from build123d import *

# Parameters (mm, degrees)
EXTRUDE_1_DEPTH = 0.5
SKETCH_2_W      = 15
SKETCH_2_H      = 2
EXTRUDE_2_DEPTH = 3.6


with BuildPart() as part:
    # 草圖1 → 填料-伸長1 (new body, symmetric)
    with BuildSketch(Plane.XY):
        with BuildLine():
            Line((-17.6, 110.46), (17.6, 110.46))
            ThreePointArc((17.6, 110.46), (26.056997103, 106.956997103), (29.56, 98.5))
            Line((29.56, 98.5), (29.56, -103.764581662))
            ThreePointArc((29.56, -103.764581662), (24.409428177, -108.417234577), (17.675642482, -110.1))
            Line((17.675642482, -110.1), (-17.524357518, -110.1))
            ThreePointArc((-17.524357518, -110.1), (-24.32498645, -108.419421277), (-29.56, -103.764581662))
            Line((-29.56, -103.764581662), (-29.56, 98.5))
            ThreePointArc((-29.56, 98.5), (-26.056997103, 106.956997103), (-17.6, 110.46))
        make_face()
    extrude(amount=EXTRUDE_1_DEPTH, both=True)

    # 草圖2 → 填料-伸長2 (add)
    with BuildSketch(Plane.XZ.offset(110.1)):
        with Locations((0, -1.5)):
            Rectangle(SKETCH_2_W, SKETCH_2_H)
        with Locations((0, 1.5)):
            Rectangle(SKETCH_2_W, SKETCH_2_H)
    extrude(amount=-EXTRUDE_2_DEPTH)


solid = part.part
Geometry: final body of the model. Coordinates: model frame, mm. Give positions to 0.01 mm unless a question says otherwise; leave off trailing zeros. Order: outer loops, then holes, each group sorted by start corner. A loop starts at its lowest first (then second) coordinate and runs counter-clockwise, first axis right, second up. Notation, with made-up numbers: (-20.5, 1) - (-1.5, 1) arc R18 cw to (-1.5, 30) - close; hole circle Ø10 at (-19.75, 67). An arc over 180 degrees is marked (long way). Use CSV: the item, a comma, the result in double quotes.
1. Section query A-A (x = -4). Output: boundary loops of the cut face in (y, z).
Answers below:
outline,"(-110.1, -2.5) - (-106.5, -2.5) - (-106.5, -0.5) - (110.46, -0.5) - (110.46, 0.5) - (-106.5, 0.5) - (-106.5, 2.5) - (-110.1, 2.5) - close"
2. Section query C-C (y = -95.5). Output: boundary loops of the cut face in (x, z), plus the area to 3 significant figures.
Answers below:
outline,"(-29.56, -0.5) - (29.56, -0.5) - (29.56, 0.5) - (-29.56, 0.5) - close"
area,"59.1 mm2"
3. Contact query for flat-ended pins moving along their axis: pin 1 (1 mm diameter, centred on y = -63.5, z = -1.5, fed in from +X); pin 2 (8 mm diameter, centred on x = 20.5, y = 66.5, fed in from +Z); pin 3 (1.6 mm diameter, centred on y = -108.5, z = 1, fed in from -X); pin 4 (1.6 mm diameter, centred on x = 2, z = 1.5, fed in from +Y). Output: stop coordinate, or through.
Answers below:
pin 1,"through"
pin 2,"z = 0.5"
pin 3,"x = -25.27"
pin 4,"y = -106.5"
4. Material intervals for line 1 along Z through (x, y) = (-1.5, 23.5); line 2 along Y through (x, z) = (-23.5, -0.45); line 3 along Y through (x, z) = (-21, -0.45), sorted ascending. Write a range as from..to.
Answers below:
line 1,"-0.5..0.5"
line 2,"-108.82..108.9"
line 3,"-109.68..109.97"
5. Section query B-B (z = 1.25). Output: boundary loops of the cut face in (x, y), plus the area to 3 significant figures.
Answers below:
outline,"(-7.5, -110.1) - (7.5, -110.1) - (7.5, -106.5) - (-7.5, -106.5) - close"
area,"54.0 mm2"
